For this review, take the finished solid that the model builds, in its own axes (mm). Coordinates: 2 decimals unless noted, no trailing zeros. Order: outer loops, then holes, each group sorted by start corner. A loop starts at its lowest first (then second) coordinate and runs counter-clockwise, first axis right, second up. Notation, with made-up numbers: (47.25, 71.5) -> (100.25, 71.5) arc R29 cw to (100.25, 103.5) -> close; hole circle Ø1 at (-8, -33). An arc over 180 degrees is marked (long way). Return JSON: item names as keys, results as strings. Group by question number.
Item 1: For line 1 along Z through (x, y) = (7.5, 116); line 2 along Y through (x, z) = (311, -99) (3 decimals); line 3 along Y through (x, z) = (198, -135.5), list the stretches that pass through material, from the lowest coordinate up.
Item 2: Take a section at B-B (x = 46.5). Write out the cut boundary in (y, z) (3 decimals).
Item 3: Insertion check: pin 1 (8 mm diameter, centred on y = 185, z = 5.5, fed in from +X); pin 2 (2 mm diameter, centred on x = 138.5, z = -231.5, fed in from -Y); pin 3 (18 mm diameter, centred on y = 521.5, z = -185, fed in from +X). Each pin has a flat end and moves straight along its axis. Give the tip position at first contact, or say it passes through.
Item 4: Take a section at D-D (y = 367). Write out the cut boundary in (x, z), then the cut area to 3 significant figures.
Item 5: Take a section at A-A (z = -204.5). Count the separate pieces of the cut face and the enclosed holes in it, then the cut area to 3 significant figures.
Item 6: Take a section at C-C (x = 174.5). Write out the cut boundary in (y, z) (3 decimals), then the cut area to 3 significant figures.
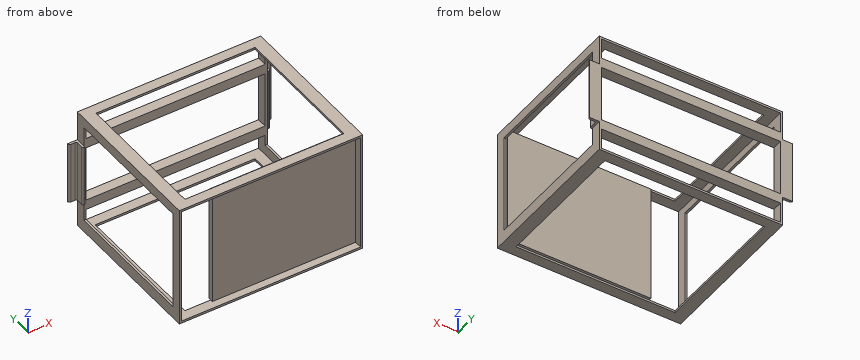
Autodesk Inventor part; units mm, degrees
ref_plane "YZ Plane" through (0, 0, 0) normal (1, 0, 0) x (0, 1, 0)
ref_plane "XZ Plane" through (0, 0, 0) normal (0, 1, 0) x (-1, 0, 0)
ref_plane "XY Plane" through (0, 0, 0) normal (0, 0, 1) x (1, 0, 0)
sketch "Boceto1" plane through (0, 0, 0) normal (0, 0, 1) x (1, 0, 0)
  line L0 (0, 0) -> (0, 544.715)
  line L1 (0, 544.715) -> (35, 544.715)
  line L2 (35, 509.715) -> (35, 0)
  line L3 (35, 0) -> (0, 0)
  line L4 (35, 544.715) -> (625, 544.715)
  line L5 (625, 544.715) -> (625, 509.715)
  line L6 (625, 509.715) -> (35, 509.715)
  line L7 (625, 509.715) -> (625, 0)
  line L8 (590, 0) -> (590, 509.715)
  line L9 (590, 0) -> (625, 0)
  line L10 (590, 0) -> (625, 0)
  line L11 (590, 509.715) -> (590, 0)
  line L12 (35, 0) -> (590, 0)
  line L13 (590, 0) -> (590, 35)
  line L14 (590, 35) -> (35, 35)
  line L15 (35, 544.715) -> (35, 509.715)
  line L16 (590, 509.715) -> (590, 544.715)
  dimension "d0" = 544.715
  dimension "d1" = 35
  dimension "d2" = 590
  dimension "d3" = 35
  dimension "d4" = 35
  dimension "d5" = 35
extrude "Extrusión1" add sketch "Boceto1" along normal blind 7.5 contours L0 L1 L15 L2 L3 | L2 L14 L8 L12 | L4 L16 L6 L15 | L8 L6 L7 L9 | L4 L5 L6 L16
ref_plane "Plano de trabajo1" through (0, 0, -617.5) normal (0, 0, -1) x (-1, 0, 0)
sketch "Boceto6" plane through (625, 0, 0) normal (1, 0, 0) x (0, 0, -1)
  line L0 (0, 0) -> (-7.5, 0)
  line L1 (-7.5, 0) -> (412.5, 0)
  line L2 (412.5, 0) -> (412.5, 544.715)
  line L3 (-7.5, 544.715) -> (-7.5, 0)
  line L4 (412.5, 544.715) -> (-7.5, 544.715)
  line L5 (-7.5, 544.715) -> (-7.5, 0)
  line L6 (-7.5, 544.715) -> (-7.5, 509.715)
  line L7 (-7.5, 509.715) -> (377.5, 509.715)
  line L8 (377.5, 509.715) -> (377.5, 35)
  line L9 (377.5, 35) -> (27.5, 35)
  line L10 (27.5, 35) -> (27.5, 509.715)
  dimension "d28" = 420
  dimension "d29" = 544.715
  dimension "d30" = 35
  dimension "d31" = 385
  dimension "d32" = 474.715
  dimension "d33" = 350
extrude "Extrusión5" add sketch "Boceto6" along normal blind 7.5
sketch "Boceto7" plane through (625, 0, -412.5) normal (0, 0, -1) x (-1, 0, 0)
  line L0 (625, 544.715) -> (-7.5, 544.715)
  line L1 (-7.5, 544.715) -> (625, 544.715)
  line L2 (625, 544.715) -> (625, 0)
  line L3 (625, 0) -> (-7.5, 0)
  line L4 (625, 0) -> (-7.5, 0)
  line L5 (-7.5, 0) -> (-7.5, 544.715)
  line L6 (-7.5, 544.715) -> (-7.5, 0)
  line L7 (-7.5, 544.715) -> (-7.5, 509.715)
  line L8 (35, 509.715) -> (593, 509.715)
  line L9 (35, 35) -> (590, 35)
  line L10 (593, 509.715) -> (590, 35)
  line L11 (590, 35) -> (35, 35)
  line L12 (35, 35) -> (35, 509.715)
  dimension "d36" = 35
  dimension "d37" = 600.5
extrude "Extrusión6" add sketch "Boceto7" along normal blind 7.5
sketch "Boceto8" plane through (0, 0, -412.5) normal (-1, 0, 0) x (0, 0, 1)
  line L0 (420, 544.715) -> (-7.5, 544.715)
  line L1 (-7.5, 544.715) -> (420, 544.715)
  line L2 (420, 544.715) -> (420, 0)
  line L3 (420, 544.715) -> (420, 0)
  line L4 (420, 0) -> (-7.5, 0)
  line L5 (412.5, 0) -> (0, 0)
  line L6 (-7.5, 0) -> (-7.5, 544.715)
  line L7 (-7.5, 35) -> (-7.5, 509.715)
  line L8 (-7.5, 544.715) -> (-7.5, 509.715)
  line L9 (385, 509.715) -> (385, 35)
  line L10 (35, 509.715) -> (385, 509.715)
  line L11 (385, 509.715) -> (385, 35)
  line L12 (35, 35) -> (35, 509.715)
  line L13 (385, 35) -> (35, 35)
  line L14 (35, 35) -> (35, 509.715)
  point P0 (144.8076, 0)
  point P1 (0, 415.0504)
  dimension "d40" = 35
extrude "Extrusión7" add sketch "Boceto8" along normal blind 7.5
sketch "Boceto9" plane through (632.5, 544.715, 7.5) normal (0, 1, 0) x (1, 0, 0)
  line L0 (-640, 0) -> (0, 0)
  line L1 (-640, 0) -> (-640, 80)
  line L2 (-640, 0) -> (-640, 427.5)
  line L3 (-640, 80) -> (0, 80)
  line L4 (0, 80) -> (0, 115)
  line L5 (0, 115) -> (-640, 115)
  line L6 (-640, 115) -> (-640, 80)
  line L7 (0, 427.5) -> (-640, 427.5)
  line L8 (-640, 427.5) -> (-640, 347.5)
  line L9 (-640, 347.5) -> (0, 347.5)
  line L10 (0, 347.5) -> (0, 312.5)
  line L11 (0, 35) -> (0, 385)
  line L12 (0, 312.5) -> (-640, 312.5)
  line L13 (-640, 312.5) -> (-640, 347.5)
  point P0 (-632.5, 7.5)
  dimension "d43" = 80
  dimension "d44" = 640
  dimension "d45" = 35
  dimension "d46" = 640
  dimension "d47" = 80
  dimension "d48" = 640
  dimension "d49" = 35
  dimension "d50" = 640
extrude "Extrusión8" add sketch "Boceto9" against normal blind 35 contours L2 L5 L4 L3 | L2 L9 L10 L12
sketch "Boceto10" plane through (632.5, 0, 0) normal (1, 0, 0) x (0, 0, -1)
  line L0 (-7.5, 544.715) -> (-7.5, 0)
  line L1 (412.5, 544.715) -> (-7.5, 544.715)
  line L2 (-7.5, 544.715) -> (107.5, 544.715)
  line L3 (107.5, 544.715) -> (97.5, 544.715)
  line L4 (-7.5, 544.715) -> (420, 544.715)
  line L5 (97.5, 544.715) -> (97.5, 504.715)
  line L6 (420, 544.715) -> (420, 0)
  line L7 (420, 544.715) -> (315, 544.715)
  line L8 (315, 544.715) -> (315, 504.715)
  line L9 (315, 504.715) -> (97.5, 504.715)
  line L10 (97.5, 544.715) -> (315, 544.715)
  point P0 (0, 0)
  point P1 (305, 544.715)
  dimension "d53" = 115
  dimension "d54" = 10
  dimension "d55" = 40
  dimension "d56" = 105
extrude "Extrusión9" add sketch "Boceto10" along normal blind 7.5
sketch "Boceto11" plane through (632.5, 504.715, -97.5) normal (0, 0, 1) x (1, 0, 0)
  line L0 (0, 40) -> (7.5, 40)
  line L1 (7.5, 40) -> (7.5, 32.5)
  line L2 (7.5, 40) -> (7.5, 0)
  line L3 (7.5, 0) -> (7.5, 40)
  line L4 (0, 40) -> (35, 40)
  line L5 (35, 40) -> (35, 32.5)
  line L6 (35, 32.5) -> (7.5, 32.5)
  line L7 (7.5, 32.5) -> (0, 32.5)
  line L8 (0, 5) -> (0, 40)
  line L9 (0, 32.5) -> (0, 40)
  point P0 (-632.5, -504.715)
  dimension "d59" = 7.5
  dimension "d64" = 35
extrude "Extrusión10" add sketch "Boceto11" against normal blind 217.5
fillet "Empalme1" radius 7.5 1 edges at (667.5, 537.215, -206.25)
fillet "Empalme2" radius 5 1 edges at (640, 537.215, -206.25)
fillet "Empalme3" radius 5 1 edges at (640, 504.715, -206.25)
sketch "Boceto14" plane through (-7.5, 0, -412.5) normal (-1, 0, 0) x (0, 0, 1)
  line L0 (-7.5, 544.715) -> (-7.5, 0)
  line L1 (97.5, 544.715) -> (-7.5, 544.715)
  line L2 (-7.5, 544.715) -> (97.5, 544.715)
  line L3 (97.5, 544.715) -> (97.5, 504.715)
  line L4 (97.5, 504.715) -> (315, 504.715)
  line L5 (315, 504.715) -> (315, 544.715)
  line L6 (315, 544.715) -> (97.5, 544.715)
  point P0 (412.5, 0)
  point P1 (0, 544.715)
  dimension "d76" = 105
  dimension "d77" = 40
  dimension "d78" = 217.5
extrude "Extrusión11" add sketch "Boceto14" along normal blind 7.5
sketch "Boceto15" plane through (-7.5, 504.715, -315) normal (0, 0, -1) x (-1, 0, 0)
  line L0 (0, 40) -> (0, 5)
  line L1 (0, 40) -> (35, 40)
  line L2 (35, 40) -> (35, 32.5)
  line L3 (35, 32.5) -> (0, 32.5)
  point P0 (-7.5, -504.715)
  dimension "d81" = 35
  dimension "d82" = 7.5
extrude "Extrusión12" add sketch "Boceto15" against normal blind 217.5
fillet "Empalme4" radius 7.5 1 edges at (-42.5, 537.215, -206.25)
fillet "Empalme5" radius 5 1 edges at (-15, 537.215, -206.25)
fillet "Empalme6" radius 5 1 edges at (-15, 504.715, -206.25)
sketch "Boceto18" plane through (35, 35, -412.5) normal (0, 1, 0) x (1, 0, 0)
  line L0 (-35, 0) -> (590, 0)
  line L1 (590, 0) -> (550, 0)
  line L2 (550, 0) -> (490, 0)
  line L3 (490, 0) -> (90, 0)
  line L4 (90, 0) -> (90, -412.5)
  line L5 (590, -412.5) -> (-35, -412.5)
  line L6 (90, -412.5) -> (590, -412.5)
  line L7 (590, -412.5) -> (590, 0)
  line L8 (590, -412.5) -> (590, 0)
  line L9 (590, 0) -> (90, 0)
  point P0 (590, -144.8076)
  dimension "d90" = 40
  dimension "d91" = 60
  dimension "d92" = 400
extrude "Extrusión13" add sketch "Boceto18" along normal mid plane 17.5
properties part number "mesa" material "Hierro, fundido"
Findings below:
{
 "1": {"line 1": "z = -420 to -412.5, 0 to 7.5", "line 2": "y = 26.25 to 43.75, 509.715 to 544.715", "line 3": "y = 26.25 to 43.75"},
 "2": {"outline": "(0, -420) -> (35, -420) -> (35, -412.5) -> (0, -412.5) -> close; (0, 0) -> (35, 0) -> (35, 7.5) -> (0, 7.5) -> close; (509.715, -420) -> (544.715, -420) -> (544.715, -412.5) -> (509.715, -412.5) -> close; (509.715, -340) -> (544.715, -340) -> (544.715, -305) -> (509.715, -305) -> close; (509.715, -107.5) -> (544.715, -107.5) -> (544.715, -72.5) -> (509.715, -72.5) -> close; (509.715, 0) -> (544.715, 0) -> (544.715, 7.5) -> (509.715, 7.5) -> close"},
 "3": {"pin 1": "stops at x = 632.5", "pin 2": "stops at y = 26.25", "pin 3": "stops at x = 640"},
 "4": {"outline": "(-7.5, -420) -> (32.9, -420) -> (32.9, -412.5) -> (0, -412.5) -> (0, -377.5) -> (-7.5, -377.5) -> close; (-7.5, -27.5) -> (0, -27.5) -> (0, 0) -> (35, 0) -> (35, 7.5) -> (-7.5, 7.5) -> close; (590, -420) -> (632.5, -420) -> (632.5, -377.5) -> (625, -377.5) -> (625, -412.5) -> (590, -412.5) -> close; (590, 0) -> (625, 0) -> (625, -27.5) -> (632.5, -27.5) -> (632.5, 7.5) -> (590, 7.5) -> close", "area": "2,200 mm2"},
 "5": {"separate pieces": "4", "enclosed holes": "0", "area": "10,800 mm2"},
 "6": {"outline": "(0, -420) -> (35, -420) -> (35, -412.5) -> (43.75, -412.5) -> (43.75, 0) -> (35, 0) -> (35, 7.5) -> (0, 7.5) -> (0, 0) -> (26.25, 0) -> (26.25, -412.5) -> (0, -412.5) -> close; (509.715, -420) -> (544.715, -420) -> (544.715, -412.5) -> (509.715, -412.5) -> close; (509.715, -340) -> (544.715, -340) -> (544.715, -305) -> (509.715, -305) -> close; (509.715, -107.5) -> (544.715, -107.5) -> (544.715, -72.5) -> (509.715, -72.5) -> close; (509.715, 0) -> (544.715, 0) -> (544.715, 7.5) -> (509.715, 7.5) -> close", "area": "10,700 mm2"}
}
